Can you work these out from the model? Positions are in its coordinate system, mm. Face numbers are marked on the shaded views. A direction names the side the tool comes from. Round coordinates to 2 decimals unless told otherwise and drop trailing zeros. Write each loop counter-clockwise with the first axis right and the second up, starting at its lowest first coordinate (ties: lowest second). Pieces come first, ordered by that corner, then holes. Notation, with made-up numbers: M -4,65.25 L 17,65.25 A13 cw 17,87.25 Z; hole C -19,72 d2. An arc over 180 degrees is marked long. Answer as a JSON object with one key per item and string values. Group by question number.
1) Suppose I cut it at D-D, the plane y = -5. Write out the boundary of the cut face in (x, z).
2) I'm going to push flat-ended pins straight in: pin 1 Ø4 at (x, y) = (-5, -5) entering from +Z; pin 2 Ø5 at (x, z) = (-5, 1.5) entering from +Y; pin 3 Ø2 at (x, z) = (3, -42.5) entering from +Y. Where does each tip first touch, or does it pass through?
3) Suppose I cut it at A-A, the plane y = 0. Write out the boundary of the cut face in (x, z) (3 decimals), and give its area (3 significant figures).
4) On a 3-axis mill with a long thin cutter (end or side, diameter ignored), from which of +Z, -Z, +X, -X, +Y, -Y can I reach the whole of each face in a straight line? I mean the marked faces 1, 2 and 3. Say none if no direction works.
5) Please list where these lines run through material, in increasing order: L1, parallel to Z at x = -1.25, y = -4; L2, parallel to Z at x = -4.75, y = -5; L3, parallel to Y at x = -5, z = -24. Write a range as [from, to].
6) Suppose I cut it at C-C, the plane z = -13. Write out the boundary of the cut face in (x, y).
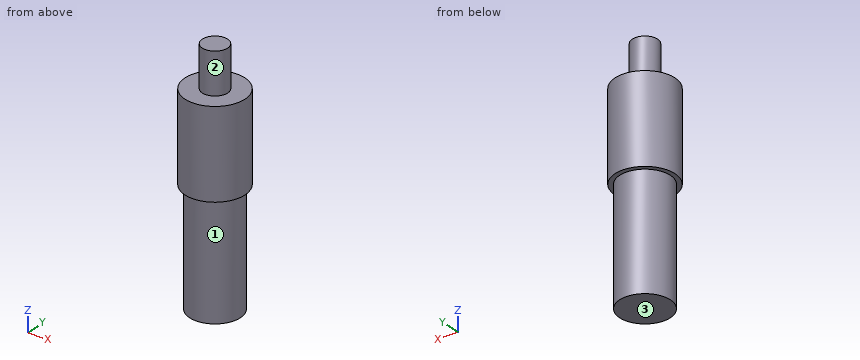
from build123d import *

# Parameters (mm, degrees)
F0_W   = 3.175
F0_H   = 10.3124
F0_W_2 = 6.35
F0_H_2 = 28.575


with BuildPart() as f1:
    # F0 (on Front) → F1 (revolve)
    with BuildSketch(Plane.XZ):
        with Locations((-1.5875, 5.1562)):
            Rectangle(F0_W, F0_H)
        Polygon((0, -21.9964), (0, 0), (-3.175, 0), (-7.5057, 0), (-7.5057, -21.9964), (-6.35, -21.9964), align=None)
        with Locations((-3.175, -36.2839)):
            Rectangle(F0_W_2, F0_H_2)
    revolve(axis=Axis((0, 0, 5.1562), (0, 0, 1)))


solid = f1.part
Results:
{
 "1": {"outline": "M -5.6,-22 L -3.91,-22 L -3.91,-50.57 L 3.91,-50.57 L 3.91,-22 L 5.6,-22 L 5.6,0 L -5.6,0 Z"},
 "2": {"pin 1": "z = 0", "pin 2": "y = 6.88", "pin 3": "y = 6.03"},
 "3": {"outline": "M -7.506,-21.996 L -6.35,-21.996 L -6.35,-50.571 L 6.35,-50.571 L 6.35,-21.996 L 7.506,-21.996 L 7.506,0 L 3.175,0 L 3.175,10.312 L -3.175,10.312 L -3.175,0 L -7.506,0 Z", "area": "759 mm^2"},
 "4": {"face 1": "-Z", "face 2": "+Z", "face 3": "-Z, +X, -X, +Y, -Y"},
 "5": {"L1": "[-50.57, 0]", "L2": "[-22, 0]", "L3": "[-3.91, 3.91]"},
 "6": {"outline": "C 0,0 d15.01"}
}
